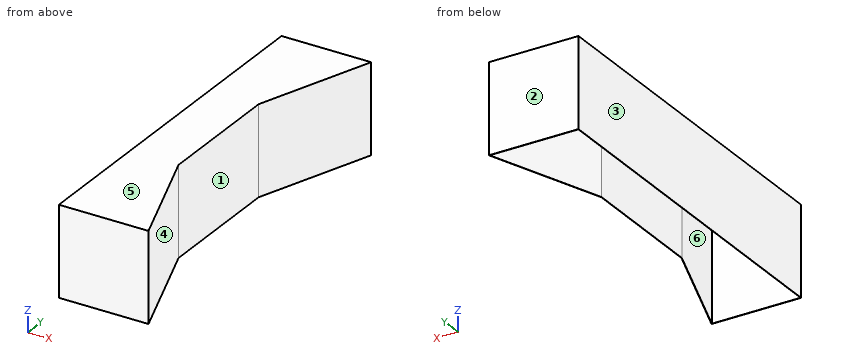
```python
from build123d import *

# Parameters (mm, degrees)
SKETCH1_W           = 1000
SKETCH1_H           = 250
BOSS_EXTRUDE1_DEPTH = 250
CUT_EXTRUDE1_DEPTH  = 573.821961869
SHELL1_T            = -1


with BuildPart() as part:
    # Sketch1 → Boss-Extrude1 (new body)
    with BuildSketch(Plane(origin=(0, 0, 0), x_dir=(0, 1, 0), z_dir=(0, 0, 1))):
        Rectangle(SKETCH1_W, SKETCH1_H)
    extrude(amount=BOSS_EXTRUDE1_DEPTH)

    # Sketch2 → Cut-Extrude1 (cut, through all)
    with BuildSketch(Plane(origin=(0, 0, 250), x_dir=(0, -1, 0), z_dir=(0, 0, 1))):
        Polygon((-500, 125), (-180, 10.108747069), (180, 10.108747069), (500, 125), align=None)
    extrude(amount=-CUT_EXTRUDE1_DEPTH, mode=Mode.SUBTRACT)

    # Shell1
    shell1_openings = [part.faces().sort_by_distance(p)[0] for p in [
        (-34.803159923, 0, 0),
    ]]
    offset(amount=SHELL1_T, openings=shell1_openings, kind=Kind.INTERSECTION)


solid = part.part
```
Geometry check sheet. Reference: the model listing, model coordinates, mm. Face numbers are marked on the shaded views. A direction names the side the tool comes from. Coordinates: 2 decimals unless noted, no trailing zeros. Order: outer loops, then holes, each group sorted by start corner. A loop starts at its lowest first (then second) coordinate and runs counter-clockwise, first axis right, second up.
Item 1: Section check B-B (x = -53). Enter the section's corners in (y, z), plus the area to 3 significant figures.
Item 2: Tool access check on the marked faces 4, 5 and 6. Record the directions out of +Z, -Z, +X, -X, +Y, -Y that give a thin tool (end or side, any length) a straight path to the whole face; none if there is none.
Item 3: Section check A-A (z = 209). Enter the section's corners in (x, y).
Item 4: Mould release check, pull along Y, two halves, no side actions. Record for the marked faces 1, 2 and 3: released by +Y, released by -Y, zero draft, split by the parting line, or undercut.
Item 5: Depth check by flat-ended pin: pin 1 (8 mm diameter, centred on y = -312.5, z = 123.5, fed in from +X); pin 2 (8 mm diameter, centred on y = 379.5, z = 50.5, fed in from +X); pin 3 (12 mm diameter, centred on x = -82, y = 201, fed in from -Z). Enter the tip coordinate at first touch or a pass-through.
Item 6: Section check C-C (y = -28). Enter the section's corners in (x, z).
Item 7: Scan lines: line 1 along X through (y, z) = (-180, 232); line 2 along Y through (x, z) = (3, 15); line 3 along Z through (x, y) = (-40, 140.5). Record each from-to range of solid material in increasing order.
Item 8: Section check D-D (x = 66). Enter the section's corners in (y, z).
Check sheet entries:
1. outline: (-500, 0) - (-499, 0) - (-499, 249) - (499, 249) - (499, 0) - (500, 0) - (500, 250) - (-500, 250) - close
1. area: 1,500 mm2
2. face 4: +Z, -Z, +X
2. face 5: +Z, +X, -X, +Y, -Y
2. face 6: -Z
3. outline: (-125, -500) - (125, -500) - (10.11, -180) - (10.11, 180) - (125, 500) - (-125, 500) - close; hole (-124, -499) - (123.58, -499) - (9.11, -180.17) - (9.11, 180.17) - (123.58, 499) - (-124, 499) - close
4. face 1: undercut
4. face 2: released by +Y
4. face 3: zero draft
5. pin 1: stops at x = 59.12
5. pin 2: stops at x = 83.17
5. pin 3: stops at z = 249
6. outline: (-125, 0) - (-124, 0) - (-124, 249) - (9.11, 249) - (9.11, 0) - (10.11, 0) - (10.11, 250) - (-125, 250) - close
7. line 1: x = -125 to -124, 9.11 to 10.11
7. line 2: y = -500 to -499, 499 to 500
7. line 3: z = 249 to 250
8. outline: (-500, 0) - (-499, 0) - (-499, 249) - (-338.63, 249) - (-338.63, 0) - (-335.67, 0) - (-335.67, 250) - (-500, 250) - close; (335.67, 0) - (338.63, 0) - (338.63, 249) - (499, 249) - (499, 0) - (500, 0) - (500, 250) - (335.67, 250) - close
